Source: CAD feature listing. Evaluate the final solid. Frame: model axes, mm. A direction names the side the tool comes from. Round coordinates to 2 decimals unless told otherwise and drop trailing zeros. Order: outer loops, then holes, each group sorted by start corner. A loop starts at its lowest first (then second) coordinate and runs counter-clockwise, first axis right, second up. Notation, with made-up numbers: (-6.75, -30.5) - (37.25, -30.5) arc R27 ccw to (37.25, -14.5) - close; hole circle Ø4 at (76, 69). An arc over 180 degrees is marked (long way). Return JSON: item names as keys, results as strings. Group by question number.
1) Contact query for flat-ended pins moving along their axis: P1, Ø2, axis at y = 0.5, z = -3, coming from the -X side; P2, Ø3, axis at x = 2, y = -1.5, coming from the -Z side. Output: stop coordinate, or through.
2) Section A-A, the plane y = 0. Return loops of the section in (x, z).
3) Mould query, pull axis Y, two halves, no side actions, for faces 1 (the flat face through (0, 3, 0)), 2 (the cylindrical face through (2.26, -0.39, 0.87)), 3 (the flat face through (8, 0, 1)). Classes: pulls with the +Y half, pulls with the -Y half, needs draft (parallel to the pull), parting line crosses it, or undercut.
4) Section D-D, the plane x = -5. Return loops of the section in (y, z), plus the area to 3 significant figures.
5) Access query for faces 4 (the flat face through (1, 0, -2)), 5 (the flat face through (4, -2, -4.9)), 6 (the flat face through (-4, 0, -6.5)). Directions: +Z, -Z, +X, -X, +Y, -Y. A direction counts if a zero-diameter tool reaches every point of the face in a straight line with its end or side. Return the directions, or none.
6) Section B-B, the plane x = 3.5. Return loops of the section in (y, z), plus the area to 3 significant figures.
7) Section C-C, the plane z = 2.75. Return loops of the section in (x, y).
8) Ray query, line 1 (Y direction, x = 3.5, z = 3.5); line 2 (Z direction, x = 4.5, y = 1.75); line 3 (X direction, y = 0, z = 0). Return the intervals inside material, ascending. Write a range as from..to.
```python
from build123d import *

# Parameters (mm, degrees)
PAD_DEPTH       = 3
SKETCH001_R     = 1.3
POCKET_DEPTH    = 11.4
SKETCH002_R     = 1.3
POCKET001_DEPTH = 9
CHAMFER_SIZE    = 0.5


with BuildPart() as part:
    # Sketch → Pad (new body, symmetric)
    with BuildSketch(Plane.XZ):
        Polygon((-8, 1.5), (-3, 6.5), (8, 6.5), (8, -4.9), (-1, -4.9), (-1, -6.5), (-8, -6.5), align=None)
    extrude(amount=PAD_DEPTH, both=True)

    # Sketch001 → Pocket (cut)
    with BuildSketch(Plane(origin=(0, 0, 6.5), x_dir=(-1, 0, 0), z_dir=(0, 0, 1))):
        with Locations((-3.5, 0)):
            Circle(SKETCH001_R)
    extrude(amount=-POCKET_DEPTH, mode=Mode.SUBTRACT)

    # Sketch002 → Pocket001 (cut)
    with BuildSketch(Plane(origin=(-8, 0, 0), x_dir=(0, 0, -1), z_dir=(-1, 0, 0))):
        with Locations((2.5, 0)):
            Circle(SKETCH002_R)
    extrude(amount=-POCKET001_DEPTH, mode=Mode.SUBTRACT)

    # Chamfer
    chamfer_edges = [part.edges().sort_by_distance(p)[0] for p in [
        (-8, 0, -1.2),
        (4.8, 0, 6.5),
        (4.8, 0, -4.9),
    ]]
    chamfer(chamfer_edges, length=CHAMFER_SIZE)


solid = part.part
```
Geometry check:
{
 "1": {"P1": "x = -7.91", "P2": "z = -4.9"},
 "2": {"outline": "(-8, -6.5) - (-1, -6.5) - (-1, -4.9) - (1.7, -4.9) - (2.2, -4.4) - (2.2, 6) - (1.7, 6.5) - (-3, 6.5) - (-8, 1.5) - (-8, -0.7) - (-7.5, -1.2) - (1, -1.2) - (1, -3.8) - (-7.5, -3.8) - (-8, -4.3) - close; (4.8, -4.4) - (5.3, -4.9) - (8, -4.9) - (8, 6.5) - (5.3, 6.5) - (4.8, 6) - close"},
 "3": {"face 1": "pulls with the +Y half", "face 2": "undercut", "face 3": "needs draft"},
 "4": {"outline": "(-3, -6.5) - (3, -6.5) - (3, 4.5) - (-3, 4.5) - close; hole circle Ø2.6 at (0, -2.5)", "area": "60.7 mm2"},
 "5": {"face 4": "-X", "face 5": "-Z, +X, +Y, -Y", "face 6": "-Z, +X, -X, +Y, -Y"},
 "6": {"outline": "(-3, -4.9) - (-1.8, -4.9) - (-1.3, -4.4) - (-1.3, 6) - (-1.8, 6.5) - (-3, 6.5) - close; (1.3, -4.4) - (1.8, -4.9) - (3, -4.9) - (3, 6.5) - (1.8, 6.5) - (1.3, 6) - close", "area": "38.3 mm2"},
 "7": {"outline": "(-6.75, -3) - (8, -3) - (8, 3) - (-6.75, 3) - close; hole circle Ø2.6 at (3.5, 0)"},
 "8": {"line 1": "-3..-1.3, 1.3..3", "line 2": "-4.9..6.5", "line 3": "-8..2.2, 4.8..8"}
}
